from build123d import *

# Parameters (mm, degrees)
BOSS_EXTRUDE1_DEPTH            = 3
BOSS_EXTRUDE1_DEPTH_BACK       = 7
BOSS_EXTRUDE2_DEPTH            = 3
BOSS_EXTRUDE2_DEPTH_BACK       = 7
SKETCH1_3_W                    = 65.055522872
SKETCH1_3_H                    = 5
CUT_EXTRUDE1_REACH             = 79.455
SKETCH2_R                      = 2
CUT_EXTRUDE2_REACH             = 62.059
CUT_EXTRUDE2_DIRECTION_2_REACH = 62.059
FILLET4_R                      = 5.5
CUT_EXTRUDE3_REACH             = 83.998
SKETCH4_R                      = 2


with BuildPart() as part:
    # Sketch1 → Boss-Extrude1 (new, two sides: drawn at the far end of the back side and taken through both)
    with BuildSketch(Plane.XY.offset(-BOSS_EXTRUDE1_DEPTH_BACK)):
        Polygon((5, 24.943962348), (-5, 24.943962348), (-21.080707518, -45), (21.383633098, -45), align=None)
    extrude(amount=BOSS_EXTRUDE1_DEPTH + BOSS_EXTRUDE1_DEPTH_BACK)

    # Sketch1_3 → Boss-Extrude2 (add, two sides: drawn at the far end of the back side and taken through both)
    with BuildSketch(Plane.XY.offset(-BOSS_EXTRUDE2_DEPTH_BACK)):
        with Locations((0, -47.5)):
            Rectangle(SKETCH1_3_W, SKETCH1_3_H)
    extrude(amount=BOSS_EXTRUDE2_DEPTH + BOSS_EXTRUDE2_DEPTH_BACK)

    # Sketch2 → Cut-Extrude1 (cut, up to next)
    with BuildSketch(Plane(origin=(0, -45, 0), x_dir=(1, 0, 0), z_dir=(0, 1, 0)), mode=Mode.PRIVATE) as cut_extrude1_sk1:
        with Locations(Location((-27.527761436, 2, 0), (0, 0, 270))):
            Circle(SKETCH2_R)
    cut_extrude1_tool1 = extrude(cut_extrude1_sk1.sketch, amount=-CUT_EXTRUDE1_REACH, mode=Mode.PRIVATE) & part.part
    # Sketch2 → Cut-Extrude1 (cut, up to next)
    with BuildSketch(Plane(origin=(0, -45, 0), x_dir=(1, 0, 0), z_dir=(0, 1, 0)), mode=Mode.PRIVATE) as cut_extrude1_sk2:
        with Locations(Location((27.527761436, 2, 0), (0, 0, 270))):
            Circle(SKETCH2_R)
    cut_extrude1_tool2 = extrude(cut_extrude1_sk2.sketch, amount=-CUT_EXTRUDE1_REACH, mode=Mode.PRIVATE) & part.part
    add(cut_extrude1_tool1.solids().sort_by_distance((-27.527761, -45, -2))[0], mode=Mode.SUBTRACT)
    add(cut_extrude1_tool2.solids().sort_by_distance((27.527761, -45, -2))[0], mode=Mode.SUBTRACT)

    # Sketch3 → Cut-Extrude2 (cut, up to next)
    with BuildSketch(Plane.XY, mode=Mode.PRIVATE) as cut_extrude2_sk1:
        Polygon((-4.467725682, 4.943962348), (4.549449769, 4.943962348), (16.248294489, -45), (-15.95026433, -45), align=None)
    cut_extrude2_tool1 = extrude(cut_extrude2_sk1.sketch, amount=-CUT_EXTRUDE2_REACH, mode=Mode.PRIVATE) & part.part
    add(cut_extrude2_tool1.solids().sort_by_distance((0.105077, -24.709767, 0))[0], mode=Mode.SUBTRACT)

    # Sketch3 → Cut-Extrude2 direction 2 (cut, up to next)
    with BuildSketch(Plane.XY, mode=Mode.PRIVATE) as cut_extrude2_direction_2_sk1:
        Polygon((-4.467725682, 4.943962348), (4.549449769, 4.943962348), (16.248294489, -45), (-15.95026433, -45), align=None)
    cut_extrude2_direction_2_tool1 = extrude(cut_extrude2_direction_2_sk1.sketch, amount=CUT_EXTRUDE2_DIRECTION_2_REACH, mode=Mode.PRIVATE) & part.part
    add(cut_extrude2_direction_2_tool1.solids().sort_by_distance((0.105077, -24.709767, 0))[0], mode=Mode.SUBTRACT)

    # Fillet4
    fillet4_edges = [part.edges().sort_by_distance(p)[0] for p in [
        (-4.467725682, 4.943962348, -2),
        (-15.95026433, -45, -2),
        (16.248294489, -45, -2),
        (4.549449769, 4.943962348, -2),
    ]]
    fillet(fillet4_edges, radius=FILLET4_R)

    # Sketch4 → Cut-Extrude3 (cut, up to next)
    with BuildSketch(Plane(origin=(0, 24.943962348, 0), x_dir=(1, 0, 0), z_dir=(0, 1, 0)), mode=Mode.PRIVATE) as cut_extrude3_sk1:
        with Locations(Location((0, 2, 0), (0, 0, 270))):
            Circle(SKETCH4_R)
    cut_extrude3_tool1 = extrude(cut_extrude3_sk1.sketch, amount=-CUT_EXTRUDE3_REACH, mode=Mode.PRIVATE) & part.part
    add(cut_extrude3_tool1.solids().sort_by_distance((0, 24.943962, -2))[0], mode=Mode.SUBTRACT)


solid = part.part
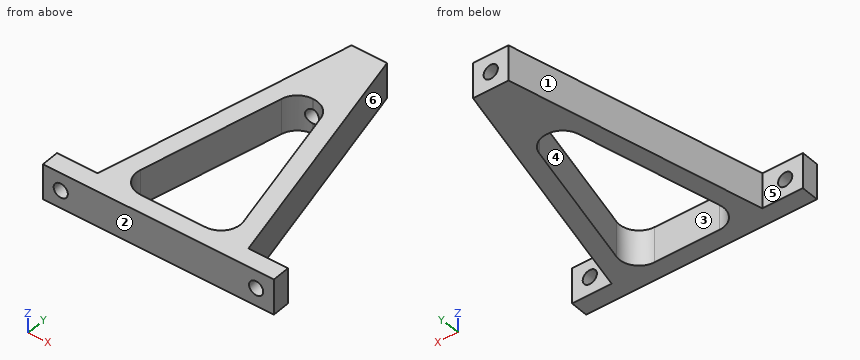
Can you work these out from the model? Positions are in its coordinate system, mm. Face numbers are marked on the shaded views. A direction names the side the tool comes from. Give positions to 0.01 mm unless a question says otherwise; leave off trailing zeros. Order: outer loops, then holes, each group sorted by start corner. A loop starts at its lowest first (then second) coordinate and runs counter-clockwise, first axis right, second up. Notation, with made-up numbers: M 19,84 L 42,84 A9 cw 42,101 Z; hole C 66.5,11.25 d8. An arc over 180 degrees is marked long. Use a Markdown table: item, result. Add a question column.
Item 1: For the marked faces 4, 5 and 6, which set-ups out of +Z, -Z, +X, -X, +Y, -Y let a thin tool reach every point of the face, with its end or its side?
Item 2: Suppose I cut it at A-A (z = 1.25). List the corners of the cut face in (x, y) for me, then the cut area to 3 significant figures.
Item 3: Suppose I cut it at D-D (x = -16.5). List the corners of the cut face in (y, z) for me.
Item 4: Suppose I cut it at B-B (y = 2.5). List the corners of the cut face in (x, z) for me, then the cut area to 3 significant figures.
Item 5: We'd pull the mould along Y, two halves only. Please class the marked faces 1, 2 and 3: +Y half, -Y half, draft (parallel to the pull), parting line (faces both ways), or undercut.
Item 6: Suppose I cut it at C-C (y = -43). List the corners of the cut face in (x, z) for me, then the cut area to 3 significant figures.
Item 7: If I drill on L1, parallel to X at y = -48.5, z = -2; L2, parallel to Z at x = 0, y = 15.5; L3, parallel to X at y = 14.5, z = -1.5, over which ranges is the centre line in solid material (lowest first)? Write a range as [from, to].
Item 8: Will these pins go through, and if not, where does the flat tip stop? pin 1 (4 mm diameter, centred on y = -34.5, z = -2, fed in from +X); pin 2 (2 mm diameter, centred on y = 15, z = -1, fed in from +X); pin 3 (5 mm diameter, centred on x = 25, z = 0, fed in from +Y).
Answer sheet:
| question | item | result |
|---|---|---|
| 1 | face 4 | +Z, -Z |
| 1 | face 5 | +Z, -Z, -X, +Y |
| 1 | face 6 | +Z, -Z, +X, +Y |
| 2 | outline | M -32.53,-50 L 32.53,-50 L 32.53,-45 L 21.38,-45 L 5,24.94 L -5,24.94 L -21.08,-45 L -32.53,-45 Z; hole M -14.4,-38.27 A5.5 ccw -9.04,-45 L 9.31,-45 A5.5 ccw 14.67,-38.25 L 5.54,0.7 A5.5 ccw 0.19,4.94 L -0.09,4.94 A5.5 ccw -5.45,0.68 Z |
| 2 | area | 1,160 mm² |
| 3 | outline | M -50,-7 L -25.08,-7 L -25.08,3 L -50,3 Z |
| 4 | outline | M -10.16,-7 L -4.66,-7 L -4.66,3 L -10.16,3 Z; M 4.76,-7 L 10.26,-7 L 10.26,3 L 4.76,3 Z |
| 4 | area | 110 mm² |
| 5 | face 1 | +Y half |
| 5 | face 2 | -Y half |
| 5 | face 3 | undercut |
| 6 | outline | M -20.62,-7 L -13.28,-7 L -13.28,3 L -20.62,3 Z; M 13.55,-7 L 20.92,-7 L 20.92,3 L 13.55,3 Z |
| 6 | area | 147 mm² |
| 7 | L1 | x = [-32.53, -29.53], [-25.53, 25.53], [29.53, 32.53] |
| 7 | L2 | z = [-7, -4], [0, 3] |
| 7 | L3 | x = [-7.4, -1.94], [1.94, 7.45] |
| 8 | pin 1 | stops at x = 19.39 |
| 8 | pin 2 | stops at x = 7.56 |
| 8 | pin 3 | stops at y = -45 |
